from build123d import *

# Parameters (mm, degrees)
BOSS_EXTRUDE1_DEPTH                             = 6.35
SKETCH2_R                                       = 14.2875
CUT_EXTRUDE1_DEPTH                              = 98.395421479
CBORE_FOR_10_SOCKET_HEAD_CAP_SCREW1_D           = 5.1054
CBORE_FOR_10_SOCKET_HEAD_CAP_SCREW1_CBORE_D     = 9.525
CBORE_FOR_10_SOCKET_HEAD_CAP_SCREW1_CBORE_DEPTH = 4.826
F_1_4_CLEARANCE_HOLE1_D                         = 6.7564


with BuildPart() as part:
    # Sketch1 → Boss-Extrude1 (new body)
    with BuildSketch(Plane(origin=(0, 0, 0), x_dir=(0, 0, -1), z_dir=(1, 0, 0))):
        with BuildLine():
            Line((52.649677831, 50.8), (76.2, 50.8))
            Line((76.2, 50.8), (76.2, 0))
            Line((76.2, 0), (52.649677831, 0))
            ThreePointArc((52.649677831, 0), (49.171639591, -1.037208832), (46.829806699, -3.81))
            ThreePointArc((46.829806699, -3.81), (38.1, -9.525), (29.370193301, -3.81))
            ThreePointArc((29.370193301, -3.81), (27.028360409, -1.037208832), (23.550322169, 0))
            Line((23.550322169, 0), (0, 0))
            Line((0, 0), (0, 50.8))
            Line((0, 50.8), (23.550322169, 50.8))
            ThreePointArc((23.550322169, 50.8), (27.028360409, 51.837208832), (29.370193301, 54.61))
            ThreePointArc((29.370193301, 54.61), (38.1, 60.325), (46.829806699, 54.61))
            ThreePointArc((46.829806699, 54.61), (49.171639591, 51.837208832), (52.649677831, 50.8))
        make_face()
    extrude(amount=BOSS_EXTRUDE1_DEPTH)

    # Sketch2 → Cut-Extrude1 (cut, through all)
    with BuildSketch(Plane(origin=(6.35, 0, 0), x_dir=(0, 0, -1), z_dir=(1, 0, 0))):
        with Locations((38.1, 25.4)):
            Circle(SKETCH2_R)
    extrude(amount=-CUT_EXTRUDE1_DEPTH, mode=Mode.SUBTRACT)

    # CBORE for #10 Socket Head Cap Screw1 (through all)
    with Locations(Plane.ZY):
        with Locations((-63.5, 25.4), (-38.1, 50.8), (-12.7, 25.4), (-38.1, 0)):
            CounterBoreHole(CBORE_FOR_10_SOCKET_HEAD_CAP_SCREW1_D / 2, CBORE_FOR_10_SOCKET_HEAD_CAP_SCREW1_CBORE_D / 2, CBORE_FOR_10_SOCKET_HEAD_CAP_SCREW1_CBORE_DEPTH)

    # 1/4 Clearance Hole1 (through all)
    with Locations(Plane(origin=(6.35, 0, 0), x_dir=(0, 0, -1), z_dir=(1, 0, 0))):
        with Locations((9.661126973, 43.174295642), (65.884030556, 43.174295642), (65.884030556, 8.467644678), (9.661126973, 8.467644678)):
            Hole(F_1_4_CLEARANCE_HOLE1_D / 2)


solid = part.part
Model file for the job. Use its own axes, mm. A direction names the side the tool comes from. Coordinates: 2 decimals unless noted, no trailing zeros. Write each loop counter-clockwise with the first axis right and the second up, starting at its lowest first coordinate (ties: lowest second). Pieces come first, ordered by that corner, then holes. Notation, with made-up numbers: (-34.5, 16) -> (-22.5, 16) arc R19 cw to (-22.5, 43) -> close; hole circle Ø7 at (-33.5, 16.25). An arc over 180 degrees is marked (long way). One line per item, written item: value. Start each with the question number.
1) Pull direction Z, two halves, no side cores. Call faces 4 (the face through (3.13, 51.81, -26.99)), 5 (the face through (3, 50.8, -64)), 6 (the face through (5.599, 0.767, -40.535)), 7 (the face through (3.131, 51.866, -49.129)): +Z half, -Z half, draft (parallel to the pull), parting line (faces both ways), or undercut.
2) Flat gauge pins, fed straight in: pin 1 Ø8 at (y, z) = (50.8, -38.1) entering from -X; pin 2 Ø2 at (x, y) = (3, 53) entering from +Z; pin 3 Ø3 at (x, z) = (3.5, -17) entering from -Y; pin 4 Ø23 at (y, z) = (25.4, -38.1) entering from +X. Where does each tip first touch, or does it go through?
3) Slice it at D-D on z = -22.5. Write the cut outline in (x, y).
4) Slice it at C-C on y = 13.5. Write the cut outline in (x, z).
5) Slice it at B-B on x = 3.25. Count the separate pieces of the cut face and the enclosed holes in it, then the cut area to 3 significant figures.
6) Probe probe 1 along Y at (x, z) = (1.95, -38.1) (1 decimal); probe 2 along Z at (x, y) = (4.5, 6); probe 3 along Y at (x, z) = (1.75, -63). List the from-to ranges inside material, lowest first.
7) Slice it at A-A on y = 25.4. Write the cut outline in (x, z).
8) Which spindle directions (+Z, -Z, +X, -X, +Y, -Y) get a long thin tool onto all of the face, cutting with end or side? Do faces 1 (the face through (3, 0, -65)), 2 (the face through (3, 0, -12)), 3 (the face through (2.379, 51.009, -42.858)). Say none if no direction does.
Answers follow:
1. face 4: +Z half
1. face 5: draft
1. face 6: undercut
1. face 7: -Z half
2. pin 1: x = 4.83
2. pin 2: z = -27.27
2. pin 3: y = 0
2. pin 4: through
3. outline: (0, 0) -> (6.35, 0) -> (6.35, 50.8) -> (0, 50.8) -> close
4. outline: (0, -76.2) -> (6.35, -76.2) -> (6.35, -46.01) -> (0, -46.01) -> close; (0, -30.19) -> (6.35, -30.19) -> (6.35, 0) -> (0, 0) -> close
5. separate pieces: 1
5. enclosed holes: 9
5. area: 3,100 mm2
6. probe 1: -9.5 to -4.8, 4.8 to 11.1, 39.7 to 46, 55.6 to 60.3
6. probe 2: -76.2 to -68.19, -63.58 to -11.97, -7.35 to 0
6. probe 3: 0 to 6.71, 10.23 to 20.66, 30.14 to 41.42, 44.93 to 50.8
7. outline: (0, -76.2) -> (6.35, -76.2) -> (6.35, -66.05) -> (4.83, -66.05) -> (4.83, -68.26) -> (0, -68.26) -> close; (0, -58.74) -> (4.83, -58.74) -> (4.83, -60.95) -> (6.35, -60.95) -> (6.35, -52.39) -> (0, -52.39) -> close; (0, -23.81) -> (6.35, -23.81) -> (6.35, -15.25) -> (4.83, -15.25) -> (4.83, -17.46) -> (0, -17.46) -> close; (0, -7.94) -> (4.83, -7.94) -> (4.83, -10.15) -> (6.35, -10.15) -> (6.35, 0) -> (0, 0) -> close
8. face 1: -Z, +X, -X, -Y
8. face 2: +Z, +X, -X, -Y
8. face 3: -X
